The listing builds one solid part. Answer for the finished solid, in the listing's coordinates (mm). Give positions to 0.01 mm unless a question says otherwise; leave off trailing zeros. Order: outer loops, then holes, each group sorted by start corner. A loop starts at its lowest first (then second) coordinate and runs counter-clockwise, first axis right, second up.
```python
from build123d import *

# Parameters (mm, degrees)
SKETCH1_R             = 14
SKETCH1_R_2           = 7
BOSS_EXTRUDE1_DEPTH   = 0.6
F_2_0MM_DOWEL_HOLE1_D = 2
CIRPATTERN1_COUNT     = 8


with BuildPart() as part:
    # Sketch1 → Boss-Extrude1 (new body, symmetric)
    with BuildSketch(Plane(origin=(0, 0, 0), x_dir=(1, 0, 0), z_dir=(0, 1, 0))):
        Circle(SKETCH1_R)
        Circle(SKETCH1_R_2, mode=Mode.SUBTRACT)
    extrude(amount=BOSS_EXTRUDE1_DEPTH, both=True)

    # Ø2.0mm Dowel Hole1 (through all)
    with Locations(Plane(origin=(0, 0.6, 0), x_dir=(1, 0, 0), z_dir=(0, 1, 0))):
        with Locations((0, 11)):
            f_2_0mm_dowel_hole1 = Hole(F_2_0MM_DOWEL_HOLE1_D / 2)

    # CirPattern1: Ø2.0mm Dowel Hole1 ×8 about axis
    cirpattern1_axis = Axis((0, 0, 0), (0, 1, 0))
    for i in range(1, CIRPATTERN1_COUNT):
        add(f_2_0mm_dowel_hole1.rotate(cirpattern1_axis, i * 360 / CIRPATTERN1_COUNT), mode=Mode.SUBTRACT)


solid = part.part
```
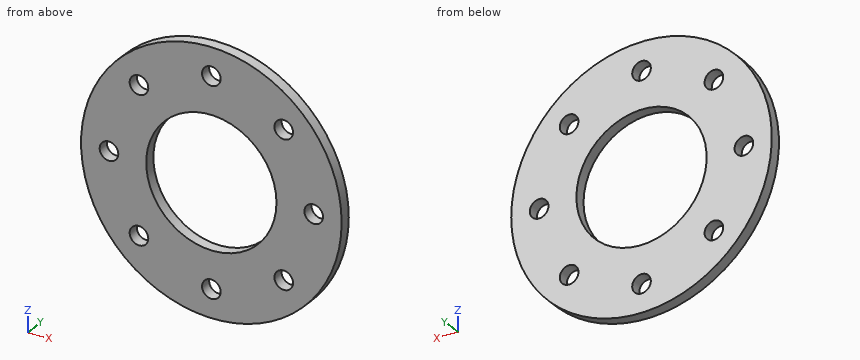
1) Find section C-C (y = -0.25). Count the separate pieces of the cut face and the enclosed holes in it, then the cut area to 3 significant figures.
Geometry says:
separate pieces: 1
enclosed holes: 9
area: 437 mm2
2) Straight lines are drawn through the part: probe 1 along Z at (x, y) = (0, -0.2); probe 2 along Z at (x, y) = (7.5, 0.3). For each, find the intervals that lie inside material, in ascending order.
Geometry says:
probe 1: z = -14 to -12, -10 to -7, 7 to 10, 12 to 14
probe 2: z = -11.82 to -8.74, -6.82 to 6.82, 8.74 to 11.82
3) Find section A-A (z = -3). Write down the section's boundary in (x, y), then the cut area to 3 significant figures.
Geometry says:
outline: (-13.67, -0.6) - (-6.32, -0.6) - (-6.32, 0.6) - (-13.67, 0.6) - close; (6.32, -0.6) - (13.67, -0.6) - (13.67, 0.6) - (6.32, 0.6) - close
area: 17.6 mm2
4) Find section B-B (x = -11). Write down the section's boundary in (y, z).
Geometry says:
outline: (-0.6, -8.66) - (0.6, -8.66) - (0.6, -1) - (-0.6, -1) - close; (-0.6, 1) - (0.6, 1) - (0.6, 8.66) - (-0.6, 8.66) - close
5) Find section D-D (x = -7.5). Write down the section's boundary in (y, z), then the cut area to 3 significant figures.
Geometry says:
outline: (-0.6, -11.82) - (0.6, -11.82) - (0.6, -8.74) - (-0.6, -8.74) - close; (-0.6, -6.82) - (0.6, -6.82) - (0.6, 6.82) - (-0.6, 6.82) - close; (-0.6, 8.74) - (0.6, 8.74) - (0.6, 11.82) - (-0.6, 11.82) - close
area: 23.8 mm2
